Verification items for the finished model (mm, model axes). Face numbers are marked on the shaded views. A direction names the side the tool comes from. Coordinates: 2 decimals unless noted, no trailing zeros. Loops run counter-clockwise (first coordinate to the right, second up) from the corner with the lowest first, then second, coordinate; pieces in that order, holes last. Notation, with made-up numbers: (62, 57) - (86, 57) arc R22 ccw to (86, 91) - close; hole circle Ø9 at (25.5, 87). An arc over 180 degrees is marked (long way). Answer as CSV lines item,"result". Start each with the question number.
1. Cross-section at D-D (z = 0). State how many separate pieces and enclosed holes the cut face has, plus the area to 3 significant figures.
2. Material ranges on line 1 (X direction, y = -0.5, z = -0.25); line 2 (Z direction, x = 0, y = 0.35); line 3 (Z direction, x = 40, y = -5), recorded low to high. Write a range as [from, to].
3. Gauge pin test, flat ends, axial feed: P1, Ø4, axis at x = 28, z = 1.5, coming from the -Y side; P2, Ø2.5, axis at x = 38, z = 0, coming from the +Y side; P3, Ø2, axis at y = -1, z = -2, coming from the +X side. Record the tip position at first contact, or that the pin passes through.
4. Cross-section at B-B (x = 0). Enter the section's corners in (y, z), plus the area to 4 significant figures.
5. Cross-section at A-A (y = -3.5). Enter the section's corners in (x, z), plus the area to 3 significant figures.
6. Cross-section at C-C (x = 40). Enter the section's corners in (y, z).
7. Set-up check for the marked faces 1 and 2: record each of +Z, -Z, +X, -X, +Y, -Y from which the full face is reachable in a straight line by a thin tool's end or side.
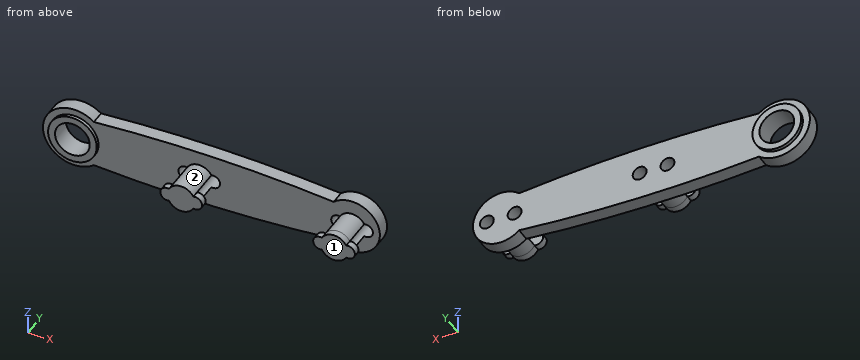
```python
from build123d import *

# Parameters (mm, degrees)
F1_DEPTH  = 1
F2_R      = 3.5
F3_DEPTH  = 1.5
F4_R      = 2.5
F5_DEPTH  = 3.001
F6_R      = 2
F7_DEPTH  = 5
F9_DEPTH  = 1
F10_R     = 1
F11_DEPTH = 6


with BuildPart() as f1:
    # F0 (on Front) → F1 (new body, symmetric)
    with BuildSketch(Plane.XZ):
        with BuildLine():
            ThreePointArc((37.3542486889, 3), (20.1018882017, 3.9785151955), (2.8284271247, 3.5))
            ThreePointArc((2.8284271247, 3.5), (-4.5, 0), (2.8284271247, -3.5))
            ThreePointArc((2.8284271247, -3.5), (20.1018882017, -3.9785151955), (37.3542486889, -3))
            ThreePointArc((37.3542486889, -3), (44, 0), (37.3542486889, 3))
        make_face()
    extrude(amount=F1_DEPTH, both=True)

    # F2 (on Front) → F3 (join, symmetric)
    with BuildSketch(Plane.XZ):
        Circle(F2_R)
    extrude(amount=F3_DEPTH, both=True)

    # F4 (on face) → F5 (cut, through all)
    with BuildSketch(Plane.XZ.offset(1.5)):
        Circle(F4_R)
    extrude(amount=-F5_DEPTH, mode=Mode.SUBTRACT)

    # F6 (on face) → F7 (join)
    with BuildSketch(Plane.XZ.offset(1)):
        with Locations((18, 0)):
            Circle(F6_R)
        with Locations((40, 0)):
            Circle(F6_R)
    extrude(amount=F7_DEPTH)

    # F8 (on face) → F9 (join)
    with BuildSketch(Plane.XZ.offset(6)):
        with BuildLine():
            ThreePointArc((16.25, -0.9682458366), (16, 0), (16.25, 0.9682458366))
            ThreePointArc((16.25, 0.9682458366), (15, 0), (16.25, -0.9682458366))
        make_face()
        with BuildLine():
            ThreePointArc((19.75, -0.9682458366), (21, 0), (19.75, 0.9682458366))
            ThreePointArc((19.75, 0.9682458366), (19.9364916731, 0.5), (20, 0))
            ThreePointArc((20, 0), (19.9364916731, -0.5), (19.75, -0.9682458366))
        make_face()
        with BuildLine():
            ThreePointArc((41.75, -0.9682458366), (43, 0), (41.75, 0.9682458366))
            ThreePointArc((41.75, 0.9682458366), (40, 2), (38.25, 0.9682458366))
            ThreePointArc((38.25, 0.9682458366), (37, 0), (38.25, -0.9682458366))
            ThreePointArc((38.25, -0.9682458366), (40, -2), (41.75, -0.9682458366))
        make_face()
        with BuildLine():
            ThreePointArc((20, 0), (19.9364916731, 0.5), (19.75, 0.9682458366))
            ThreePointArc((19.75, 0.9682458366), (18, 2), (16.25, 0.9682458366))
            ThreePointArc((16.25, 0.9682458366), (16, 0), (16.25, -0.9682458366))
            ThreePointArc((16.25, -0.9682458366), (18, -2), (19.75, -0.9682458366))
            ThreePointArc((19.75, -0.9682458366), (19.9364916731, -0.5), (20, 0))
        make_face()
    extrude(amount=-F9_DEPTH)

    # F10 (on face) → F11 (cut, through all)
    with BuildSketch(Plane(origin=(0, 1, 0), x_dir=(-1, 0, 0), z_dir=(0, 1, 0))):
        with Locations((-42, 0)):
            Circle(F10_R)
        with Locations((-38, 0)):
            Circle(F10_R)
        with Locations((-20, 0)):
            Circle(F10_R)
        with Locations((-16, 0)):
            Circle(F10_R)
    extrude(amount=-F11_DEPTH, mode=Mode.SUBTRACT)


solid = f1.part
```
Values follow:
1,separate pieces,"6"
1,enclosed holes,"0"
1,area,"101 mm²"
2,line 1,"x = [-4.49, -2.49], [2.49, 15.03], [16.97, 19.03], [20.97, 37.03], [38.97, 41.03], [42.97, 43.99]"
2,line 2,"z = [-4.5, -2.5], [2.5, 4.5]"
2,line 3,"z = [-2, 2]"
3,P1,"stops at y = -1"
3,P2,"stops at y = 1"
3,P3,"stops at x = 43.87"
4,outline,"(-1.5, -3.5) - (-1, -3.5) - (-1, -4.5) - (1, -4.5) - (1, -3.5) - (1.5, -3.5) - (1.5, -2.5) - (-1.5, -2.5) - close; (-1.5, 2.5) - (1.5, 2.5) - (1.5, 3.5) - (1, 3.5) - (1, 4.5) - (-1, 4.5) - (-1, 3.5) - (-1.5, 3.5) - close"
4,area,"10.00 mm²"
5,outline,"(16.25, -0.97) arc R2 ccw to (19.75, -0.97) arc R1 cw to (19.75, 0.97) arc R2 ccw to (16.25, 0.97) arc R1 cw to start; (38.25, -0.97) arc R2 ccw to (41.75, -0.97) arc R1 cw to (41.75, 0.97) arc R2 ccw to (38.25, 0.97) arc R1 cw to start"
5,area,"19.5 mm²"
6,outline,"(-6, -2) - (-1, -2) - (-1, -4) - (1, -4) - (1, 4) - (-1, 4) - (-1, 2) - (-6, 2) - close"
7,face 1,"+Z, -Z, +X, -X, -Y"
7,face 2,"+Z, -Y"
